from build123d import *

# Parameters (mm, degrees)
CROQUIS1_R                   = 2.1
SALIENTE_EXTRUIR1_DEPTH      = 3
TALADRO_DE_MARGEN_PARA_M51_D = 5.5
CORTAR_EXTRUIR1_DEPTH        = 3


with BuildPart() as part:
    # Croquis1 → Saliente-Extruir1 (new body)
    with BuildSketch(Plane.XY):
        with BuildLine():
            Line((-143.5, 0), (143.5, 0))
            Line((143.5, 0), (143.5, 30))
            Line((143.5, 30), (9.355173022, 385.226719524))
            ThreePointArc((9.355173022, 385.226719524), (0, 391.693910765), (-9.355173022, 385.226719524))
            Line((-9.355173022, 385.226719524), (-143.5, 30))
            Line((-143.5, 30), (-143.5, 0))
        make_face()
        with Locations((0, 365)):
            Circle(CROQUIS1_R, mode=Mode.SUBTRACT)
        with Locations((0, 335)):
            Circle(CROQUIS1_R, mode=Mode.SUBTRACT)
    extrude(amount=SALIENTE_EXTRUIR1_DEPTH)

    # Taladro de margen para M51 (through all)
    with Locations(Plane(origin=(0, 0, 0), x_dir=(-1, 0, 0), z_dir=(0, 0, -1))):
        with Locations((-85, 15), (85, 15)):
            Hole(TALADRO_DE_MARGEN_PARA_M51_D / 2)

    # Croquis4 → Cortar-Extruir1 (cut)
    with BuildSketch(Plane(origin=(0, 0, 0), x_dir=(-1, 0, 0), z_dir=(0, 0, -1))):
        with BuildLine():
            Line((9.355173022, 250.226719524), (74.889584061, 76.686118864))
            ThreePointArc((74.889584061, 76.686118864), (73.760226731, 67.466838773), (65.534411039, 63.153310105))
            Line((65.534411039, 63.153310105), (-65.534411039, 63.153310105))
            ThreePointArc((-65.534411039, 63.153310105), (-73.760226731, 67.466838773), (-74.889584061, 76.686118864))
            Line((-74.889584061, 76.686118864), (-9.355173022, 250.226719524))
            ThreePointArc((-9.355173022, 250.226719524), (0, 256.693910765), (9.355173022, 250.226719524))
        make_face()
    extrude(amount=-CORTAR_EXTRUIR1_DEPTH, mode=Mode.SUBTRACT)


solid = part.part
Geometry check sheet. Reference: the model listing, model coordinates, mm. A direction names the side the tool comes from. Give positions to 0.01 mm unless a question says otherwise; leave off trailing zeros. Loops run counter-clockwise (first coordinate to the right, second up) from the corner with the lowest first, then second, coordinate; pieces in that order, holes last. Notation, with made-up numbers: M 29.25,-7.75 L 63.25,-7.75 A21 cw 63.25,28.25 Z; hole C 46,14.5 d7. An arc over 180 degrees is marked long. Answer as a JSON object with one key per item and string values. Group by question number.
Item 1: Gauge pin test, flat end, axial feed: pin 1 (3.5 mm diameter, centred on x = -85, y = 15, fed in from +Z). Record the tip position at first contact, or that the pin passes through.
Item 2: Sectioned sample at D-D on y = 301. Record the boundary of the cut face in (x, z).
Item 3: Sectioned sample at B-B on x = -70. Record the boundary of the cut face in (y, z).
Item 4: Access from +Z, -Z, +X, -X, +Y, -Y to the whole of each face (thin tool, end or side, straight path). Record for faces 1 (the cylindrical face through (73.683, 67.356, 1.479)), 2 (the flat face through (62, 155, 3)).
Item 5: Material ranges on L1, parallel to Y at x = 0, z = 0.8; L2, parallel to X at y = 335, z = 1.4; L3, parallel to X at y = 365, z = 2, recorded low to high.
Item 6: Mould release check, pull along X, two halves, no side actions. Record for faces 3 (the flat face through (-41.664, 164.671, 1.479)), 4 (the flat face through (62, 155, 0)), 5 (the flat face through (77.367, 205.127, 1.479)), 6 (the flat face through (-75.49, 210.1, 1.48)): pulls with the +X half, pulls with the -X half, needs draft (parallel to the pull), parting line crosses it, or undercut.
Item 7: Sectioned sample at C-C on y = 216.5. Record the boundary of the cut face in (x, z), plus the area to 3 significant figures.
Item 8: Sectioned sample at A-A on z = 1.3. Record the boundary of the cut face in (x, y).
Findings below:
{
 "1": {"pin 1": "through"},
 "2": {"outline": "M -41.16,0 L 41.16,0 L 41.16,3 L -41.16,3 Z"},
 "3": {"outline": "M 0,0 L 64.21,0 L 64.21,3 L 0,3 Z; M 89.63,0 L 224.63,0 L 224.63,3 L 89.63,3 Z"},
 "4": {"face 1": "+Z, -Z", "face 2": "+Z, +X, -X, +Y, -Y"},
 "5": {"L1": "0 to 63.15, 256.69 to 332.9, 337.1 to 362.9, 367.1 to 391.69", "L2": "-28.32 to -2.1, 2.1 to 28.32", "L3": "-16.99 to -2.1, 2.1 to 16.99"},
 "6": {"face 3": "undercut", "face 4": "needs draft", "face 5": "pulls with the +X half", "face 6": "pulls with the -X half"},
 "7": {"outline": "M -73.07,0 L -22.09,0 L -22.09,3 L -73.07,3 Z; M 22.09,0 L 73.07,0 L 73.07,3 L 22.09,3 Z", "area": "306 mm2"},
 "8": {"outline": "M -143.5,0 L 143.5,0 L 143.5,30 L 9.36,385.23 A10 ccw -9.36,385.23 L -143.5,30 Z; hole C -85,15 d5.5; hole M -74.89,76.69 A10 ccw -65.53,63.15 L 65.53,63.15 A10 ccw 74.89,76.69 L 9.36,250.23 A10 ccw -9.36,250.23 Z; hole C 0,335 d4.2; hole C 0,365 d4.2; hole C 85,15 d5.5"}
}
